Could you check a few things on this drawing? It's one solid part, dimensions in mm from its lowest x, y, z. A direction names the side the tool comes from. Round coordinates to 2 decimals unless told otherwise and drop trailing zeros. Order: outer loops, then holes, each group sorted by start corner. A loop starts at its lowest first (then second) coordinate and runs counter-clockwise, first axis right, second up. Notation, with made-up numbers: (-11, -16) -> (26, -16) arc R30 ccw to (26, 14) -> close; hole circle Ø5 at (-36, 84). An arc over 180 degrees is marked (long way). Use a Markdown table: item, result. Add a question column.
(1) If I drill on probe 1 along Y at (x, z) = (12.5, 2.15); probe 2 along Y at (x, z) = (2.25, 9.5); probe 3 along Z at (x, y) = (4, 31.5), over which ranges is the centre line in solid material (lowest first)?
(2) On a 3-axis mill with a long thin cutter (end or side, diameter ignored), from which of +Z, -Z, +X, -X, +Y, -Y can I reach the whole of each face in a straight line? I mean the marked faces 1, 2 and 3. Say none if no direction works.
(3) I want a section at A-A, the plane x = 12.5. Please give me the cut outline in (y, z), then the cut area to 3 significant figures.
(4) I want a section at C-C, the plane y = 16. Please give me the cut outline in (x, z).
(5) I want a section at B-B, the plane y = 21. Please give me the cut outline in (x, z).
(6) I want a section at D-D, the plane z = 7.5. Please give me the cut outline in (x, y), then the cut area to 3 significant figures.
(7) I'm going to push flat-ended pins straight in: P1, Ø5, axis at x = 15, y = 23, coming from the -Z side; P2, Ø12.5, axis at x = 18, y = 10.5, coming from the +Z side; P3, Ø3.5, axis at x = 1.5, z = 6.5, coming from the +Y side; P4, Ø4, axis at y = 4.5, z = 6.5, coming from the +X side. Where does each tip first touch, or does it pass through?
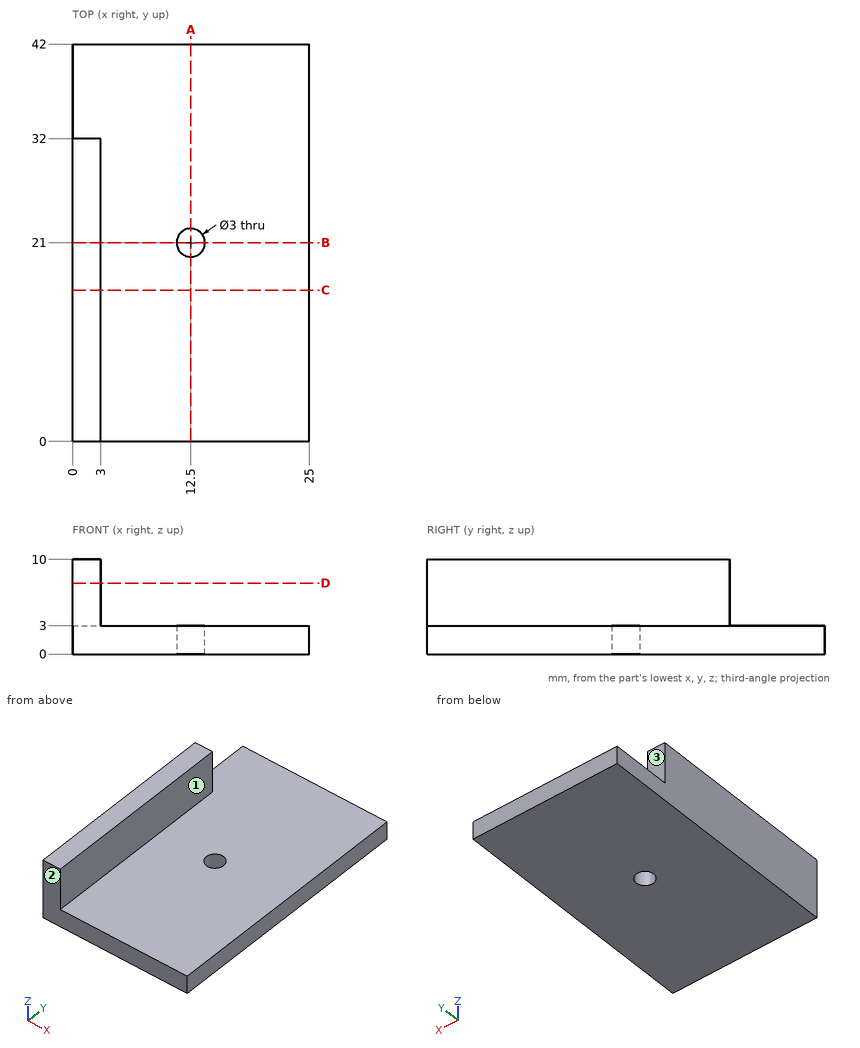
Taken from the geometry:
| question | item | result |
|---|---|---|
| 1 | probe 1 | y = 0 to 19.5, 22.5 to 42 |
| 1 | probe 2 | y = 0 to 32 |
| 1 | probe 3 | z = 0 to 3 |
| 2 | face 1 | +Z, +X, +Y, -Y |
| 2 | face 2 | +Z, -Z, +X, -X, -Y |
| 2 | face 3 | +Z, +X, -X, +Y |
| 3 | outline | (0, 0) -> (19.5, 0) -> (19.5, 3) -> (0, 3) -> close; (22.5, 0) -> (42, 0) -> (42, 3) -> (22.5, 3) -> close |
| 3 | area | 117 mm2 |
| 4 | outline | (0, 0) -> (25, 0) -> (25, 3) -> (3, 3) -> (3, 10) -> (0, 10) -> close |
| 5 | outline | (0, 0) -> (11, 0) -> (11, 3) -> (3, 3) -> (3, 10) -> (0, 10) -> close; (14, 0) -> (25, 0) -> (25, 3) -> (14, 3) -> close |
| 6 | outline | (0, 0) -> (3, 0) -> (3, 32) -> (0, 32) -> close |
| 6 | area | 96.0 mm2 |
| 7 | P1 | stops at z = 0 |
| 7 | P2 | stops at z = 3 |
| 7 | P3 | stops at y = 32 |
| 7 | P4 | stops at x = 3 |
